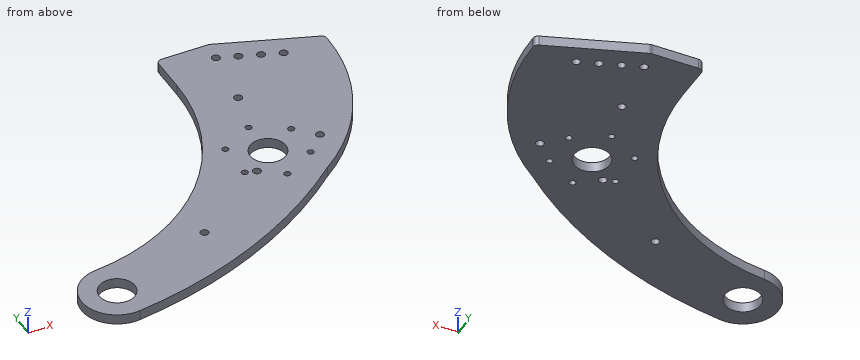
Autodesk Inventor part; units mm, degrees
ref_plane "YZ Plane" through (0, 0, 0) normal (1, 0, 0) x (0, 1, 0)
ref_plane "XZ Plane" through (0, 0, 0) normal (0, 1, 0) x (-1, 0, 0)
ref_plane "XY Plane" through (0, 0, 0) normal (0, 0, 1) x (1, 0, 0)
sketch "Sketch1" plane through (0, 0, 0) normal (0, 0, 1) x (1, 0, 0)
  line L0 (-146.05, 101.6) -> (76.2, 101.6) construction
  line L1 (76.2, 101.6) -> (76.2, 76.2) construction
  line L2 (76.2, 76.2) -> (-146.05, 76.2) construction
  line L3 (-146.05, 76.2) -> (-146.05, 101.6) construction
  circle A0 centre (-133.35, -76.2) radius 12.7 construction
  circle A1 centre (0, 0) radius 23.8125 construction
  circle A2 centre (0, 0) radius 11.1125
  circle A3 centre (0, 0) radius 36.5125 construction
  line L4 (76.2, 101.6) -> (76.2, 76.2)
  line L5 (76.2, 101.6) -> (-18.177, 101.6)
  line L6 (-18.177, 101.6) -> (-18.177, 76.2)
  circle A4 centre (-133.35, -76.2) radius 22.225 construction
  arc A5 (-135.6449, -54.0938) -> (-18.177, 76.2) centre (-149.171, 76.2) ccw
  arc A6 (-130.367, -98.2239) -> (24.2247, -27.319) centre (-169.5727, 191.233) ccw
  arc A7 (-135.6449, -54.0938) -> (-130.367, -98.2239) centre (-133.35, -76.2) ccw
  arc A8 (20.9302, -29.9181) -> (76.2, 76.2) centre (-53.3082, 76.2) ccw
  arc A9 (24.2247, -27.319) -> (30.9373, -19.3918) centre (0, 0) ccw
  line L7 (-69.85, 101.6) -> (-69.85, 76.2) construction
  line L8 (12.7, 88.9) -> (75.7926, 65.9362) construction
  line L9 (14.9394, 101.6) -> (76.2, 79.3029)
  point P0 (63.5, 88.9)
  point P1 (76.2, 88.9)
  point P2 (50.8, 88.9)
  point P3 (38.1, 88.9)
  point P4 (25.4, 88.9)
  point P5 (20.9302, -29.9181)
  point P6 (-34.5726, 11.7429)
  point P7 (22.7258, -28.6389)
  point P8 (-69.85, 88.9)
  point P9 (24.6341, 84.5563)
  point P10 (36.5682, 80.2127)
  point P11 (48.5023, 75.869)
  dimension "d0" = 25.4
  dimension "d1" = 76.2
  dimension "d2" = 222.25
  dimension "d3" = 146.05
  dimension "d4" = 25.4
  dimension "d5" = 76.2
  dimension "d7" = 12.7
  dimension "d8" = 47.625
  dimension "d9" = 22.225
  dimension "d12" = 12.7
  dimension "d17" = 12.7
  dimension "d18" = 9.525
  dimension "d19" = 292.1
  dimension "d37" = 146.05
  dimension "d38" = 63.5
  dimension "d39" = 20
  dimension "d42" = 12.7
  dimension "d47" = 12.7
extrude "Extrusion1" add sketch "Sketch1" along normal blind 6.35 contours L4 A8 A6 A7 A5 L6 L5 L9
hole "Hole1" at (36.5682, 80.2127, 0) at (48.5023, 75.869, 0) at (24.6341, 84.5563, 0) at (12.7, 88.9, 0) direction (0, 0, 1) diameter 5.1054 end through all
hole "Hole2" at (-133.35, -76.2, 0) direction (0, 0, 1) diameter 22.225 end through all
fillet "Fillet1" radius 3.175 3 edges at (76.2, 79.3029, 3.175) (14.9394, 101.6, 3.175) (-18.177, 101.6, 3.175)
sketch "Sketch3" plane through (0, 0, 6.35) normal (0, 0, 1) x (1, 0, 0)
  arc A0 (-15.002, 101.6) -> (-18.177, 98.425) centre (-15.002, 98.425) ccw construction
  line L0 (-18.177, 98.425) -> (-18.177, 76.2) construction
  arc A1 (-135.6449, -54.0938) -> (-18.177, 76.2) centre (-149.171, 76.2) ccw construction
  arc A2 (-135.6449, -54.0938) -> (-130.367, -98.2239) centre (-133.35, -76.2) ccw construction
  arc A3 (-130.367, -98.2239) -> (22.7258, -28.6389) centre (-169.5727, 191.233) ccw construction
  arc A4 (22.7258, -28.6389) -> (76.2, 76.2) centre (-53.3082, 76.2) ccw construction
  line L1 (76.2, 76.2) -> (76.2, 77.0798) construction
  arc A5 (76.2, 77.0798) -> (74.1109, 80.0633) centre (73.025, 77.0798) ccw construction
  line L2 (74.1109, 80.0633) -> (15.4654, 101.4085) construction
  arc A6 (15.4654, 101.4085) -> (14.3795, 101.6) centre (14.3795, 98.425) ccw construction
  line L3 (14.3795, 101.6) -> (-15.002, 101.6) construction
  circle A7 centre (-133.35, -76.2) radius 11.1125 construction
  circle A8 centre (24.6341, 84.5563) radius 2.5527 construction
  circle A9 centre (36.5682, 80.2127) radius 2.5527 construction
  circle A10 centre (48.5023, 75.869) radius 2.5527 construction
  circle A11 centre (12.7, 88.9) radius 2.5527 construction
  circle A12 centre (0, 0) radius 11.1125 construction
  circle A13 centre (0, 0) radius 23.8125 construction
  point P0 (0, 23.8125)
  point P1 (-20.6222, 11.9063)
  point P2 (-20.6222, -11.9062)
  point P3 (0, -23.8125)
  point P4 (20.6222, -11.9063)
  point P5 (20.6222, 11.9062)
  dimension "d49" = 47.625
  dimension "d52" = 360
hole "Hole3" at (0, 23.8125, 6.35) at (-20.6222, 11.9063, 6.35) at (-20.6222, -11.9062, 6.35) at (0, -23.8125, 6.35) at (20.6222, -11.9063, 6.35) at (20.6222, 11.9062, 6.35) direction (0, 0, -1) diameter 3.9624 end through all
sketch "Sketch6" plane through (0, 0, 6.35) normal (0, 0, 1) x (1, 0, 0)
  line L0 (14.3795, 101.6) -> (-15.002, 101.6) construction
  line L1 (-18.177, 98.425) -> (-18.177, 76.2) construction
  circle A0 centre (20.6222, -11.9063) radius 1.9812 construction
  circle A1 centre (-20.6222, -11.9062) radius 1.9812 construction
  circle A2 centre (0, 23.8125) radius 1.9812 construction
  circle A3 centre (-20.6222, 11.9063) radius 1.9812 construction
  circle A4 centre (0, -23.8125) radius 1.9812 construction
  circle A5 centre (20.6222, 11.9062) radius 1.9812 construction
  arc A6 (-15.002, 101.6) -> (-18.177, 98.425) centre (-15.002, 98.425) ccw construction
  line L2 (-18.177, 98.425) -> (-18.177, 76.2) construction
  arc A7 (-135.6449, -54.0938) -> (-18.177, 76.2) centre (-149.171, 76.2) ccw construction
  arc A8 (-135.6449, -54.0938) -> (-130.367, -98.2239) centre (-133.35, -76.2) ccw construction
  arc A9 (-130.367, -98.2239) -> (22.7258, -28.6389) centre (-169.5727, 191.233) ccw construction
  arc A10 (22.7258, -28.6389) -> (76.2, 76.2) centre (-53.3082, 76.2) ccw construction
  line L3 (76.2, 76.2) -> (76.2, 77.0798) construction
  arc A11 (76.2, 77.0798) -> (74.1109, 80.0633) centre (73.025, 77.0798) ccw construction
  line L4 (74.1109, 80.0633) -> (15.4654, 101.4085) construction
  arc A12 (15.4654, 101.4085) -> (14.3795, 101.6) centre (14.3795, 98.425) ccw construction
  line L5 (14.3795, 101.6) -> (-15.002, 101.6) construction
  circle A13 centre (-133.35, -76.2) radius 11.1125 construction
  circle A14 centre (24.6341, 84.5563) radius 2.5527 construction
  circle A15 centre (36.5682, 80.2127) radius 2.5527 construction
  circle A16 centre (48.5023, 75.869) radius 2.5527 construction
  circle A17 centre (12.7, 88.9) radius 2.5527 construction
  circle A18 centre (0, 0) radius 11.1125 construction
  circle A19 centre (-133.35, -76.2) radius 11.1125 construction
  arc A20 (-133.35, -76.2) -> (0, 0) centre (-190.0979, 177.8901) ccw construction
  point P0 (7.223, 50.8)
  point P1 (32.623, 0)
  point P2 (-65.6674, -50.8)
  point P3 (-14.0068, -13.8754)
  dimension "d76" = 50.8
  dimension "d77" = 50.8
  dimension "d78" = 25.4
  dimension "d79" = 25.4
  dimension "d91" = 260.35
  dimension "d92" = 63.5
  dimension "d93" = 25.4
hole "Hole4" at (7.223, 50.8, 6.35) at (32.623, 0, 6.35) at (-65.6674, -50.8, 6.35) at (-14.0068, -13.8754, 6.35) direction (0, 0, -1) diameter 5.1054 end through all
sketch "Sketch4" plane through (0, 0, 6.35) normal (0, 0, 1) x (1, 0, 0)
  circle A0 centre (20.6222, -11.9063) radius 1.9812 construction
  circle A1 centre (-20.6222, -11.9062) radius 1.9812 construction
  circle A2 centre (0, 23.8125) radius 1.9812 construction
  circle A3 centre (-20.6222, 11.9063) radius 1.9812 construction
  circle A4 centre (0, -23.8125) radius 1.9812 construction
  circle A5 centre (20.6222, 11.9062) radius 1.9812 construction
  arc A6 (-5.9095, 152.4) -> (-9.0845, 149.225) centre (-5.9095, 149.225) ccw construction
  line L0 (-9.0845, 149.225) -> (-9.0845, 127) construction
  arc A7 (-144.4803, -107.7629) -> (-9.0845, 127) centre (-280.3101, 127) ccw construction
  arc A8 (-144.4803, -107.7629) -> (-126.1231, -148.0172) centre (-133.35, -127) ccw construction
  arc A9 (-126.1231, -148.0172) -> (30.851, -19.5766) centre (-221.1051, 128.2089) ccw construction
  arc A10 (30.851, -19.5766) -> (76.2, 127) centre (-183.3562, 127) ccw construction
  line L1 (76.2, 127) -> (76.2, 127.8798) construction
  arc A11 (76.2, 127.8798) -> (74.1109, 130.8633) centre (73.025, 127.8798) ccw construction
  line L2 (74.1109, 130.8633) -> (15.4654, 152.2085) construction
  arc A12 (15.4654, 152.2085) -> (14.3795, 152.4) centre (14.3795, 149.225) ccw construction
  line L3 (14.3795, 152.4) -> (-5.9095, 152.4) construction
  circle A13 centre (-133.35, -127) radius 11.1125 construction
  circle A14 centre (24.6341, 135.3563) radius 2.5527 construction
  circle A15 centre (36.5682, 131.0127) radius 2.5527 construction
  circle A16 centre (48.5023, 126.669) radius 2.5527 construction
  circle A17 centre (12.7, 139.7) radius 2.5527 construction
  circle A18 centre (0, 0) radius 11.1125 construction
  circle A19 centre (0, 0) radius 30.1625 construction
  arc A20 (25.4856, -16.173) -> (69.8464, 125.6579) centre (-183.3562, 127) ccw construction
  arc A21 (-128.1879, -142.0123) -> (25.4856, -16.173) centre (-221.1051, 128.2089) ccw construction
  arc A22 (-141.3002, -113.2592) -> (-128.1879, -142.0123) centre (-133.35, -127) ccw construction
  arc A23 (-141.3002, -113.2592) -> (-2.7345, 127) centre (-280.3101, 127) ccw construction
  line L4 (-2.7345, 127) -> (-2.7345, 146.05) construction
  line L5 (-2.7345, 146.05) -> (13.8197, 146.05) construction
  line L6 (69.8464, 125.6579) -> (13.8197, 146.05) construction
  circle A24 centre (12.7, 139.7) radius 8.9027 construction
  circle A25 centre (24.6341, 84.5563) radius 2.5527 construction
  circle A26 centre (24.6341, 135.3563) radius 8.9027 construction
  circle A27 centre (36.5682, 131.0127) radius 8.9027 construction
  circle A28 centre (48.5023, 126.669) radius 8.9027 construction
  circle A29 centre (-133.35, -127) radius 17.4625 construction
  arc A30 (-18.2433, 35.5165) -> (-2.7345, 127) centre (-280.3101, 127) ccw
  arc A31 (38.1257, 4.2843) -> (69.8464, 125.6579) centre (-183.3562, 127) ccw
  arc A32 (-135.2217, -109.6381) -> (-36.2919, -5.3003) centre (-280.3101, 127) ccw
  arc A33 (-121.1415, -139.4856) -> (-135.2217, -109.6381) centre (-133.35, -127) ccw
  line L7 (-18.2433, 35.5165) -> (-7.0656, 29.3233)
  line L8 (38.1257, 4.2843) -> (28.6082, 9.5576)
  line L9 (14.5187, -33.4528) -> (7.0656, -29.3233)
  line L10 (-36.2919, -5.3003) -> (-28.6082, -9.5576)
  arc A34 (-121.1415, -139.4856) -> (14.5187, -33.4528) centre (-221.1051, 128.2089) ccw
  circle A35 centre (0, 0) radius 11.1125 construction
  arc A36 (-28.6082, -9.5576) -> (7.0656, -29.3233) centre (0, 0) ccw
  arc A37 (28.6082, 9.5576) -> (-7.0656, 29.3233) centre (0, 0) ccw
  arc A38 (40.4011, 122.9773) -> (56.5376, 130.5019) centre (48.5023, 126.669) ccw
  arc A39 (28.467, 127.321) -> (40.4011, 122.9773) centre (36.5682, 131.0127) ccw
  arc A40 (16.5329, 131.6646) -> (28.467, 127.321) centre (24.6341, 135.3563) ccw
  arc A41 (6.4602, 133.35) -> (16.5329, 131.6646) centre (12.7, 139.7) ccw
  line L11 (6.4602, 133.35) -> (-2.7345, 133.35)
  line L12 (-2.7345, 133.35) -> (-2.7345, 127)
  line L13 (69.8464, 125.6579) -> (56.5376, 130.5019)
  dimension "d62" = 6.35
  dimension "d63" = 6.35
  dimension "d64" = 6.35
  dimension "d65" = 6.35
  dimension "d66" = 6.35
  dimension "d67" = 6.35
  dimension "d68" = 22.225
  dimension "d69" = 22.225
  dimension "d70" = 12.7
  dimension "d74" = 351.8694
  dimension "d75" = 127.1124
properties part number "CL7-008" material "Polycarbonate, Smoke"
The listing builds one solid part. Answer for the finished solid, in the listing's coordinates (mm). Give positions to 0.01 mm unless a question says otherwise; leave off trailing zeros. Loops run counter-clockwise (first coordinate to the right, second up) from the corner with the lowest first, then second, coordinate; pieces in that order, holes last. Notation, with made-up numbers: M 15.25,12.25 L 45.25,12.25 A24 cw 45.25,38.25 Z; hole C -32.5,18 d10. An arc over 180 degrees is marked long. One line per item, written item: value.
1. Find the intervals of material crossed by probe 1 along X at (y, z) = (-24.5, 2.5); probe 2 along Y at (x, z) = (26, 3.5); probe 3 along X at (y, z) = (52, 0.5), in increasing order.
Found:
probe 1: -65.39 to -1.86, 1.86 to 28.13
probe 2: -26.18 to 82.4, 86.71 to 97.57
probe 3: -20.43 to 4.97, 9.48 to 73.92
2. Section B-B on z = 5 is taken. State how many separate pieces and enclosed holes the cut face has, plus the area to 3 significant figures.
Found:
separate pieces: 1
enclosed holes: 16
area: 17,300 mm^2
3. Section C-C on y = 50.8 is taken. Determine the outline of the cut face in (x, z), plus the area to 3 significant figures.
Found:
outline: M -20.66,0 L 4.67,0 L 4.67,6.35 L -20.66,6.35 Z; M 9.78,0 L 73.68,0 L 73.68,6.35 L 9.78,6.35 Z
area: 567 mm^2
4. Section A-A on y = 0 is taken. Determine the outline of the cut face in (x, z).
Found:
outline: M -42.62,0 L -11.11,0 L -11.11,6.35 L -42.62,6.35 Z; M 11.11,0 L 30.07,0 L 30.07,6.35 L 11.11,6.35 Z; M 35.18,0 L 51.41,0 L 51.41,6.35 L 35.18,6.35 Z
5. Each of these flat-tipped pins is pushed along its axis until it touches: P1, Ø1, axis at y = -11, z = 3.5, coming from the +X side; P2, Ø1, axis at y = 61, z = 4.5, coming from the -X side; P3, Ø1, axis at y = -36.5, z = 3, coming from the +X side. Where does it stop, or does it pass through?
Found:
P1: x = 42.9
P2: x = -19.12
P3: x = 13.97
6. Section D-D on x = -80 is taken. Determine the outline of the cut face in (y, z), plus the area to 3 significant figures.
Found:
outline: M -86.79,0 L -35.04,0 L -35.04,6.35 L -86.79,6.35 Z
area: 329 mm^2
